Geometry check sheet. Reference: the model listing, model coordinates, mm. A direction names the side the tool comes from. Coordinates: 2 decimals unless noted, no trailing zeros. Write each loop counter-clockwise with the first axis right and the second up, starting at its lowest first coordinate (ties: lowest second). Pieces come first, ordered by that corner, then holes. Notation, with made-up numbers: M 40,43 L 99,43 A15 cw 99,62 Z; hole C 22.25,-38.5 d8. An arc over 180 degrees is marked long. Write item = value, one per line. Start each with the question number.
```python
from build123d import *
from build123d.topology import SkipClean

# Parameters (mm, degrees)
SKETCH1_R           = 3.5
SKETCH1_R_2         = 1.5
BOSS_EXTRUDE1_DEPTH = 16.7
SKETCH4_R           = 7.5
SKETCH4_R_2         = 3.5
BOSS_EXTRUDE5_DEPTH = 2
SKETCH5_R           = 17.4
BOSS_EXTRUDE7_DEPTH = 8
BOSS_EXTRUDE8_START = -18.7
SKETCH4_2_R         = 7.5
SKETCH4_2_R_2       = 3.5
BOSS_EXTRUDE8_DEPTH = 2


with BuildPart() as part:
    # Sketch1 → Boss-Extrude1 (new body)
    with BuildSketch(Plane(origin=(0, 0, 0), x_dir=(1, 0, 0), z_dir=(0, 1, 0))):
        with BuildLine():
            Line((-32.5, -40), (32.5, -40))
            ThreePointArc((32.5, -40), (37.803300859, -37.803300859), (40, -32.5))
            Line((40, -32.5), (40, 32.5))
            ThreePointArc((40, 32.5), (37.803300859, 37.803300859), (32.5, 40))
            Line((32.5, 40), (-32.5, 40))
            ThreePointArc((-32.5, 40), (-37.803300859, 37.803300859), (-40, 32.5))
            Line((-40, 32.5), (-40, -32.5))
            ThreePointArc((-40, -32.5), (-37.803300859, -37.803300859), (-32.5, -40))
        make_face()
        with Locations(Location((32.5, 32.5, 0), (0, 0, 270))):
            Circle(SKETCH1_R, mode=Mode.SUBTRACT)
        with Locations(Location((-32.5, -32.5, 0), (0, 0, 90))):
            Circle(SKETCH1_R, mode=Mode.SUBTRACT)
        with Locations(Location((-32.5, 32.5, 0), (0, 0, 90))):
            Circle(SKETCH1_R, mode=Mode.SUBTRACT)
        with Locations(Location((32.5, -32.5, 0), (0, 0, 270))):
            Circle(SKETCH1_R, mode=Mode.SUBTRACT)
        with Locations(Location((22.600505063, -22.600505063, 0), (0, 0, 270))):
            Circle(SKETCH1_R_2, mode=Mode.SUBTRACT)
        with Locations(Location((-22.600505063, -22.600505063, 0), (0, 0, 90))):
            Circle(SKETCH1_R_2, mode=Mode.SUBTRACT)
        with Locations(Location((-22.600505063, 22.600505063, 0), (0, 0, 270))):
            Circle(SKETCH1_R_2, mode=Mode.SUBTRACT)
        with Locations(Location((22.600505063, 22.600505063, 0), (0, 0, 90))):
            Circle(SKETCH1_R_2, mode=Mode.SUBTRACT)
    extrude(amount=BOSS_EXTRUDE1_DEPTH)

    # Sketch4 → Boss-Extrude5 (add)
    # profile 1 of 4: a face of its own
    with BuildSketch(Plane(origin=(0, 16.7, 0), x_dir=(1, 0, 0), z_dir=(0, 1, 0))):
        with Locations(Location((32.5, 32.5, 0), (0, 0, 90))):
            Circle(SKETCH4_R)
        with Locations(Location((32.5, 32.5, 0), (0, 0, 90))):
            Circle(SKETCH4_R_2, mode=Mode.SUBTRACT)
    # profile 2 of 4: a face of its own
    with BuildSketch(Plane(origin=(0, 16.7, 0), x_dir=(1, 0, 0), z_dir=(0, 1, 0))):
        with Locations(Location((32.5, -32.5, 0), (0, 0, 90))):
            Circle(SKETCH4_R)
        with Locations(Location((32.5, -32.5, 0), (0, 0, 90))):
            Circle(SKETCH4_R_2, mode=Mode.SUBTRACT)
    # profile 3 of 4: a face of its own
    with BuildSketch(Plane(origin=(0, 16.7, 0), x_dir=(1, 0, 0), z_dir=(0, 1, 0))):
        with Locations(Location((-32.5, -32.5, 0), (0, 0, 90))):
            Circle(SKETCH4_R)
        with Locations(Location((-32.5, -32.5, 0), (0, 0, 90))):
            Circle(SKETCH4_R_2, mode=Mode.SUBTRACT)
    # profile 4 of 4: a face of its own
    with BuildSketch(Plane(origin=(0, 16.7, 0), x_dir=(1, 0, 0), z_dir=(0, 1, 0))):
        with Locations(Location((-32.5, 32.5, 0), (0, 0, 90))):
            Circle(SKETCH4_R)
        with Locations(Location((-32.5, 32.5, 0), (0, 0, 90))):
            Circle(SKETCH4_R_2, mode=Mode.SUBTRACT)
    extrude(amount=BOSS_EXTRUDE5_DEPTH)

    # Sketch5 → Boss-Extrude7 (add)
    with BuildSketch(Plane.XZ):
        with Locations(Location((0, 0, 0), (0, 0, 270))):
            Circle(SKETCH5_R)
    extrude(amount=BOSS_EXTRUDE7_DEPTH)

    # Sketch4<2> → Boss-Extrude8 (add)
    # profile 1 of 4: a face of its own
    with SkipClean():  # the faces are left unmerged after this step: merging them gives an invalid solid
        with BuildSketch(Plane(origin=(0, 16.7, 0), x_dir=(1, 0, 0), z_dir=(0, 1, 0)).offset(BOSS_EXTRUDE8_START)):
            with Locations(Location((32.5, 32.5, 0), (0, 0, 90))):
                Circle(SKETCH4_2_R)
            with Locations(Location((32.5, 32.5, 0), (0, 0, 90))):
                Circle(SKETCH4_2_R_2, mode=Mode.SUBTRACT)
        # profile 2 of 4: a face of its own
        with BuildSketch(Plane(origin=(0, 16.7, 0), x_dir=(1, 0, 0), z_dir=(0, 1, 0)).offset(BOSS_EXTRUDE8_START)):
            with Locations(Location((32.5, -32.5, 0), (0, 0, 90))):
                Circle(SKETCH4_2_R)
            with Locations(Location((32.5, -32.5, 0), (0, 0, 90))):
                Circle(SKETCH4_2_R_2, mode=Mode.SUBTRACT)
        # profile 3 of 4: a face of its own
        with BuildSketch(Plane(origin=(0, 16.7, 0), x_dir=(1, 0, 0), z_dir=(0, 1, 0)).offset(BOSS_EXTRUDE8_START)):
            with Locations(Location((-32.5, -32.5, 0), (0, 0, 90))):
                Circle(SKETCH4_2_R)
            with Locations(Location((-32.5, -32.5, 0), (0, 0, 90))):
                Circle(SKETCH4_2_R_2, mode=Mode.SUBTRACT)
        # profile 4 of 4: a face of its own
        with BuildSketch(Plane(origin=(0, 16.7, 0), x_dir=(1, 0, 0), z_dir=(0, 1, 0)).offset(BOSS_EXTRUDE8_START)):
            with Locations(Location((-32.5, 32.5, 0), (0, 0, 90))):
                Circle(SKETCH4_2_R)
            with Locations(Location((-32.5, 32.5, 0), (0, 0, 90))):
                Circle(SKETCH4_2_R_2, mode=Mode.SUBTRACT)
        extrude(amount=BOSS_EXTRUDE8_DEPTH)


solid = part.part
```
Q1. Cross-section at D-D on y = 4. Count the separate pieces of the cut face and the enclosed holes in it, and give its area (3 significant figures).
Q2. Set-up check for faces 5 (the face through (-1, 16.7, -1)), 6 (the face through (0, 8, -40)): record each of +Z, -Z, +X, -X, +Y, -Y from which the full face is reachable in a straight line by a thin tool's end or side.
Q3. Cross-section at A-A on z = -12. Enter the section's corners in (x, y), and give its area (3 significant figures).
Q4. Draft check along X on faces 1 (the face through (-31, -2, -36)), 2 (the face through (-1, 0, -18)), 3 (the face through (-10.6, -3.9, 13.8)), 4 (the face through (-40, 8, 0)). Enter one of: pulls with the +X half, pulls with the -X half, needs draft (parallel to the pull), parting line crosses it, or undercut.
Q5. Cross-section at C-C on z = -34. Enter the section's corners in (x, y), and give its area (3 significant figures).
Q6. Scan lines: L1, parallel to X at y = 11, z = -32.5; L2, parallel to Z at x = 32.5, y = 18.05. Record each from-to range of solid material in increasing order.
Q7. Cross-section at B-B on x = 0. Enter the section's corners in (y, z), and give its area (3 significant figures).
Q8. Gauge pin test, flat ends, axial feed: pin 1 (1.8 mm diameter, centred on x = 22.6, z = -22.6, fed in from +Y); pin 2 (16.5 mm diameter, centred on x = 31, z = 34, fed in from -Y); pin 3 (4 mm diameter, centred on x = -21.5, z = 18, fed in from -Y); pin 4 (5 mm diameter, centred on x = -22.6, z = 22.6, fed in from +Y). Record the tip position at first contact, or that the pin passes through.
Values found:
q1.separate_pieces = 1
q1.enclosed_holes = 8
q1.area = 6,170 mm²
q2.face_5 = +Y
q2.face_6 = -Z, +X, -X, +Y, -Y
q3.outline = M -40,0 L -12.6,0 L -12.6,-8 L 12.6,-8 L 12.6,0 L 40,0 L 40,16.7 L -40,16.7 Z
q3.area = 1,540 mm²
q4.face_1 = needs draft
q4.face_2 = undercut
q4.face_3 = parting line crosses it
q4.face_4 = pulls with the -X half
q5.outline = M -39.85,-2 L -35.66,-2 L -35.66,18.7 L -39.85,18.7 Z; M -29.34,-2 L -25.15,-2 L -25.15,0 L 25.15,0 L 25.15,-2 L 29.34,-2 L 29.34,18.7 L 25.15,18.7 L 25.15,16.7 L -25.15,16.7 L -25.15,18.7 L -29.34,18.7 Z; M 35.66,-2 L 39.85,-2 L 39.85,18.7 L 35.66,18.7 Z
q5.area = 1,190 mm²
q6.L1 = -40 to -36, -29 to 29, 36 to 40
q6.L2 = -40 to -36, -29 to -25, 25 to 29, 36 to 40
q7.outline = M -8,-17.4 L 0,-17.4 L 0,-40 L 16.7,-40 L 16.7,40 L 0,40 L 0,17.4 L -8,17.4 Z
q7.area = 1,610 mm²
q8.pin_1 = through
q8.pin_2 = -2
q8.pin_3 = 0
q8.pin_4 = 16.7
